Here's how the part is built. I have some questions about the finished solid (model axes, mm). Face numbers are marked on the shaded views. A direction names the side the tool comes from. Round coordinates to 2 decimals unless told otherwise and drop trailing zeros. Order: outer loops, then holes, each group sorted by start corner. A loop starts at its lowest first (then second) coordinate and runs counter-clockwise, first axis right, second up. Notation, with made-up numbers: (43, 16.25) - (81, 16.25) arc R17 cw to (81, 36.25) - close; hole circle Ø8 at (23, 34). An arc over 180 degrees is marked (long way). One line per item, written item: value.
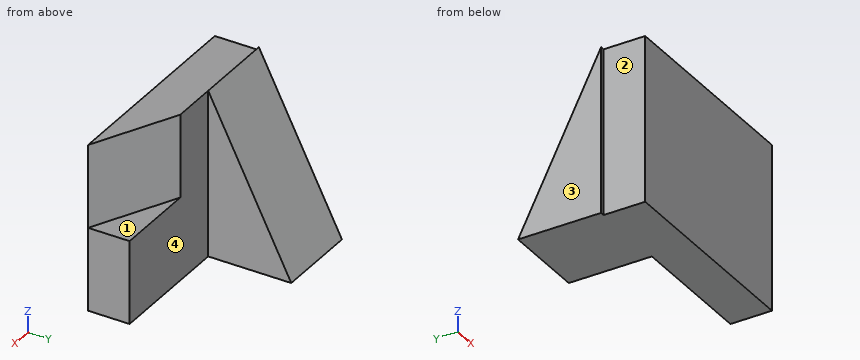
from build123d import *

# Parameters (mm, degrees)
SKETCH2_W           = 127
SKETCH2_H           = 101.6
BOSS_EXTRUDE1_DEPTH = 25.4
CUT_EXTRUDE2_DEPTH  = 50.8
BOSS_EXTRUDE2_DEPTH = 50.8


with BuildPart() as part:
    # Sketch2 → Boss-Extrude1 (new body)
    with BuildSketch(Plane(origin=(0, 0, 0), x_dir=(1, 0, 0), z_dir=(0, 1, 0))):
        with Locations((63.5, 50.8)):
            Rectangle(SKETCH2_W, SKETCH2_H)
    extrude(amount=BOSS_EXTRUDE1_DEPTH)

    # Sketch4 → Cut-Extrude2 (cut)
    with BuildSketch(Plane.XY):
        Polygon((76.2, 25.4), (127, 25.4), (127, 0), align=None)
    extrude(amount=-CUT_EXTRUDE2_DEPTH, mode=Mode.SUBTRACT)

    # Sketch5 → Boss-Extrude2 (add)
    with BuildSketch(Plane.ZY.offset(2.54)):
        Polygon((-101.6, 25.4), (0, 25.4), (-101.6, 76.2), align=None)
    extrude(amount=-BOSS_EXTRUDE2_DEPTH)


solid = part.part
Q1. If we section it at B-B, the plane x = 104: Please give me the cut outline in (y, z).
Results list:
outline: (0, -101.6) - (25.4, -101.6) - (25.4, -50.8) - (11.5, -50.8) - (11.5, 0) - (0, 0) - close
Q2. If I drill on line 1 along Y through (x, z) = (55.5, -81.5); line 2 along X through (y, z) = (27, -74); line 3 along Z through (x, y) = (79, 24.5), over which ranges is the centre line in solid material (lowest first)?
Results list:
line 1: 0 to 25.4
line 2: -2.54 to 48.26
line 3: -101.6 to -50.8
Q3. Which directions (+Z, -Z, +X, -X, +Y, -Y) give clear straight access to the entire face, cutting with the end or side of a thin tool? Please do the marked faces 1, 2, 3 and 4.
Results list:
face 1: +Z, +X, +Y
face 2: +Z, -Z, -X, -Y
face 3: +Z, -Z, -X, +Y, -Y
face 4: +Z, -Z, +X, +Y
Q4. If we section it at C-C, the plane y = 5: Please give me the cut outline in (x, z).
Results list:
outline: (0, -101.6) - (127, -101.6) - (127, -50.8) - (117, -50.8) - (117, 0) - (0, 0) - close
Q5. Will these pins go through, and if not, where does the flat tip stop? pin 1 (6 mm diameter, centred on x = 107.5, z = -75, fed in from +Y); pin 2 (12.5 mm diameter, centred on y = 14.5, z = -76, fed in from -X); pin 3 (6 mm diameter, centred on x = 46.5, z = -82, fed in from +Y).
Results list:
pin 1: y = 25.4
pin 2: x = 0
pin 3: y = 67.9
Q6. If we section it at A-A, the plane z = -60: Please give me the cut outline in (x, y), then the cut area to 3 significant figures.
Results list:
outline: (-2.54, 25.4) - (0, 25.4) - (0, 0) - (127, 0) - (127, 25.4) - (48.26, 25.4) - (48.26, 55.4) - (-2.54, 55.4) - close
area: 4,750 mm²
Q7. If we section it at D-D, the plane z = -35: Please give me the cut outline in (x, y), then the cut area to 3 significant figures.
Results list:
outline: (-2.54, 25.4) - (0, 25.4) - (0, 0) - (127, 0) - (76.2, 25.4) - (48.26, 25.4) - (48.26, 42.9) - (-2.54, 42.9) - close
area: 3,470 mm²
